```python
from build123d import *

# Parameters (mm, degrees)
SKETCH1_W               = 86.36
SKETCH1_H               = 48.26
BOSS_EXTRUDE1_DEPTH     = 3.175
CUT_EXTRUDE1_DEPTH      = 99.980593174
CUT_EXTRUDE1_DEPTH_BACK = 99.980593174
SKETCH2_R               = 2.5527
SKETCH3_R               = 2.5527
SKETCH3_R_2             = 2.54
CUT_EXTRUDE2_DEPTH      = 99.980593174
SKETCH4_R               = 2.5527
CUT_EXTRUDE3_DEPTH      = 99.980593174


with BuildPart() as part:
    # Sketch1 → Boss-Extrude1 (new body)
    with BuildSketch(Plane.XY):
        with Locations((43.18, 24.13)):
            Rectangle(SKETCH1_W, SKETCH1_H)
    extrude(amount=BOSS_EXTRUDE1_DEPTH)

    # Sketch2 → Cut-Extrude1 (cut, two sides: drawn at the far end of the back side and taken through both)
    with BuildSketch(Plane.XY.offset(3.175).offset(-CUT_EXTRUDE1_DEPTH_BACK)):
        with Locations((6.35, 36.83)):
            Circle(SKETCH2_R)
        with Locations((6.35, 11.43)):
            Circle(SKETCH2_R)
        with Locations((19.05, 36.83)):
            Circle(SKETCH2_R)
        with Locations((19.05, 11.43)):
            Circle(SKETCH2_R)
        with Locations((31.75, 36.83)):
            Circle(SKETCH2_R)
        with Locations((31.75, 11.43)):
            Circle(SKETCH2_R)
    extrude(amount=CUT_EXTRUDE1_DEPTH + CUT_EXTRUDE1_DEPTH_BACK, mode=Mode.SUBTRACT)

    # Sketch3 → Cut-Extrude2 (cut, through all)
    with BuildSketch(Plane(origin=(0, 0, 0), x_dir=(-1, 0, 0), z_dir=(0, 0, -1))):
        with Locations((-76.2, 36.83)):
            Circle(SKETCH3_R)
        with Locations((-76.2, 24.13)):
            Circle(SKETCH3_R)
        with Locations((-50.8, 36.83)):
            Circle(SKETCH3_R_2)
        with Locations((-50.8, 24.13)):
            Circle(SKETCH3_R)
    extrude(amount=-CUT_EXTRUDE2_DEPTH, mode=Mode.SUBTRACT)

    # Sketch4 → Cut-Extrude3 (cut, through all)
    with BuildSketch(Plane(origin=(0, 0, 0), x_dir=(-1, 0, 0), z_dir=(0, 0, -1))):
        with Locations((-76.2, 11.43)):
            Circle(SKETCH4_R)
        with Locations((-63.5, 11.43)):
            Circle(SKETCH4_R)
        with Locations((-50.8, 11.43)):
            Circle(SKETCH4_R)
    extrude(amount=-CUT_EXTRUDE3_DEPTH, mode=Mode.SUBTRACT)


solid = part.part
```
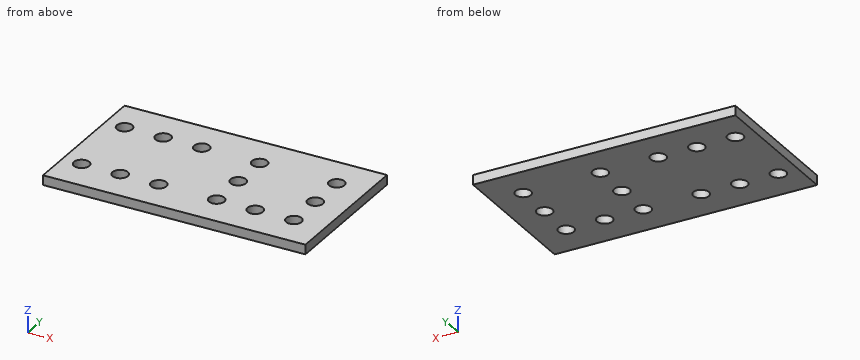
Check sheet for the modelled part. Datum: model origin and axes. Units: mm. Coordinates: 2 decimals unless noted, no trailing zeros. Write each loop counter-clockwise with the first axis right and the second up, starting at its lowest first coordinate (ties: lowest second). Pieces come first, ordered by that corner, then holes. Notation, with made-up numbers: (53.25, 84.5) - (66.25, 84.5) arc R23 cw to (66.25, 115.5) - close; hole circle Ø5 at (11.5, 29.5). An arc over 180 degrees is marked (long way). One line per question, with ' | ' between items.
Item 1: Sectioned sample at A-A on y = 36.83. Record the boundary of the cut face in (x, z) (3 decimals).
Determined:
outline: (0, 0) - (3.797, 0) - (3.797, 3.175) - (0, 3.175) - close; (8.903, 0) - (16.497, 0) - (16.497, 3.175) - (8.903, 3.175) - close; (21.603, 0) - (29.197, 0) - (29.197, 3.175) - (21.603, 3.175) - close; (34.303, 0) - (48.26, 0) - (48.26, 3.175) - (34.303, 3.175) - close; (53.34, 0) - (73.647, 0) - (73.647, 3.175) - (53.34, 3.175) - close; (78.753, 0) - (86.36, 0) - (86.36, 3.175) - (78.753, 3.175) - close
Item 2: Sectioned sample at C-C on z = 2.45. Give the number of separate pieces and of enclosed holes in the cut face, plus the area to 3 significant figures.
Determined:
separate pieces: 1 | enclosed holes: 13 | area: 3,900 mm2
Item 3: Sectioned sample at D-D on y = 24.13. Record the boundary of the cut face in (x, z) (3 decimals).
Determined:
outline: (0, 0) - (48.247, 0) - (48.247, 3.175) - (0, 3.175) - close; (53.353, 0) - (73.647, 0) - (73.647, 3.175) - (53.353, 3.175) - close; (78.753, 0) - (86.36, 0) - (86.36, 3.175) - (78.753, 3.175) - close
Item 4: Thickness scan on line 1 (Y direction, x = 31.75, z = 0.7); line 2 (Y direction, x = 50.8, z = 2.1); line 3 (X direction, y = 36.5, z = 1.2). Record the ranges inside material, lowest first. Write a range as [from, to].
Determined:
line 1: y = [0, 8.88], [13.98, 34.28], [39.38, 48.26] | line 2: y = [0, 8.88], [13.98, 21.58], [26.68, 34.29], [39.37, 48.26] | line 3: x = [0, 3.82], [8.88, 16.52], [21.58, 29.22], [34.28, 48.28], [53.32, 73.67], [78.73, 86.36]
Item 5: Gauge pin test, flat end, axial feed: P1, Ø1.5, axis at y = 33.5, z = 1.5, coming from the -X side. Record the tip position at first contact, or that the pin passes through.
Determined:
P1: stops at x = 0
Item 6: Sectioned sample at B-B on x = 63.5. Record the boundary of the cut face in (y, z) (3 decimals), plus the area to 3 significant figures.
Determined:
outline: (0, 0) - (8.877, 0) - (8.877, 3.175) - (0, 3.175) - close; (13.983, 0) - (48.26, 0) - (48.26, 3.175) - (13.983, 3.175) - close | area: 137 mm2
